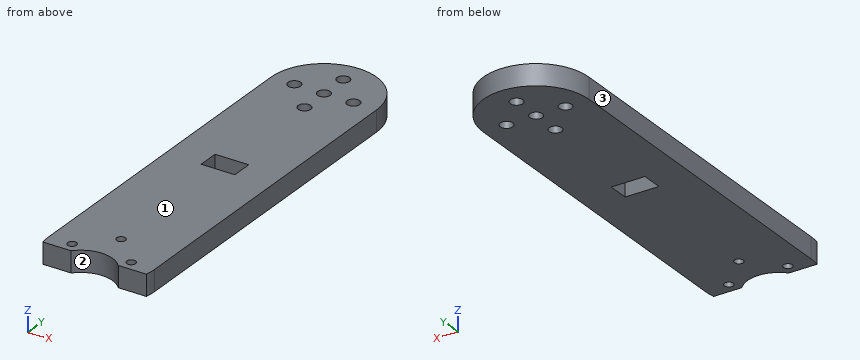
from build123d import *

# Parameters (mm, degrees)
SKETCH1_R           = 1.5
SKETCH1_R_2         = 1.493875789
SKETCH1_R_3         = 1.05
BOSS_EXTRUDE1_DEPTH = 5
SKETCH3_W           = 8
SKETCH3_H           = 5
CUT_EXTRUDE3_DEPTH  = 10
SKETCH5_R           = 7.5
SKETCH5_W           = 24.494897428
SKETCH5_H           = 10
CUT_EXTRUDE4_DEPTH  = 10


with BuildPart() as part:
    # Sketch1 → Boss-Extrude1 (new body)
    with BuildSketch(Plane.XY):
        with BuildLine():
            Line((-12.5, 0), (-12.5, -80))
            ThreePointArc((-12.5, -80), (0, -92.5), (12.5, -80))
            Line((12.5, -80), (12.5, 0))
            ThreePointArc((12.5, 0), (0, 12.5), (-12.5, 0))
        make_face()
        with Locations((0, 6.993875789)):
            Circle(SKETCH1_R, mode=Mode.SUBTRACT)
        Circle(SKETCH1_R_2, mode=Mode.SUBTRACT)
        with Locations((-7, -80)):
            Circle(SKETCH1_R_3, mode=Mode.SUBTRACT)
        with Locations((0, -73)):
            Circle(SKETCH1_R_3, mode=Mode.SUBTRACT)
        with Locations((7, -80)):
            Circle(SKETCH1_R_3, mode=Mode.SUBTRACT)
        with Locations((-6.993875789, 0)):
            Circle(SKETCH1_R, mode=Mode.SUBTRACT)
        with Locations((0, -6.993875789)):
            Circle(SKETCH1_R, mode=Mode.SUBTRACT)
        with Locations((6.993875789, 0)):
            Circle(SKETCH1_R, mode=Mode.SUBTRACT)
    extrude(amount=BOSS_EXTRUDE1_DEPTH)

    # Sketch3 → Cut-Extrude3 (cut)
    with BuildSketch(Plane.XY.offset(5)):
        with Locations((0, -35.613875789)):
            Rectangle(SKETCH3_W, SKETCH3_H)
    extrude(amount=-CUT_EXTRUDE3_DEPTH, mode=Mode.SUBTRACT)

    # Sketch5 → Cut-Extrude4 (cut)
    with BuildSketch(Plane.XY.offset(5)):
        with Locations((0, -87.5)):
            Circle(SKETCH5_R)
        with Locations((0, -87.5)):
            Rectangle(SKETCH5_W, SKETCH5_H)
    extrude(amount=-CUT_EXTRUDE4_DEPTH, mode=Mode.SUBTRACT)


solid = part.part
For this review, take the finished solid that the model builds, in its own axes (mm). Face numbers are marked on the shaded views. Give positions to 0.01 mm unless a question says otherwise; leave off trailing zeros. Loops run counter-clockwise (first coordinate to the right, second up) from the corner with the lowest first, then second, coordinate; pieces in that order, holes last.
Item 1: Take a section at C-C, the plane z = 3.3. Give the number of separate pieces and of enclosed holes in the cut face, and give its area (3 significant figures).
Item 2: Draft analysis for pull direction X (two halves, no side actions). For the marked faces 1, 2 and 3, state which applies: +X half, -X half, draft (parallel to the pull), parting line (faces both ways), or undercut.
Item 3: Take a section at D-D, the plane x = -11. State the section outline as (y, z) points.
Item 4: For line 1 along Y through (x, z) = (0, 3.45); line 2 along X through (y, z) = (-73, 3.05); line 3 along Y through (x, z) = (-0.75, 4.15), list the stretches that pass through material, from the lowest coordinate up.
Item 5: Take a section at A-A, the plane x = 0. State the section outline as (y, z) points, and give its area (3 significant figures).
Item 6: Take a section at B-B, the plane x = -7. State the section outline as (y, z) points.
Calculated:
1. separate pieces: 1
1. enclosed holes: 9
1. area: 2,200 mm2
2. face 1: draft
2. face 2: undercut
2. face 3: -X half
3. outline: (-82.5, 0) - (5.94, 0) - (5.94, 5) - (-82.5, 5) - close
4. line 1: y = -80 to -74.05, -71.95 to -38.11, -33.11 to -8.49, -5.49 to -1.49, 1.49 to 5.49, 8.49 to 12.5
4. line 2: x = -12.5 to -1.05, 1.05 to 12.5
4. line 3: y = -80.04 to -73.73, -72.27 to -38.11, -33.11 to -8.29, -5.69 to -1.29, 1.29 to 5.69, 8.29 to 12.48
5. outline: (-80, 0) - (-74.05, 0) - (-74.05, 5) - (-80, 5) - close; (-71.95, 0) - (-38.11, 0) - (-38.11, 5) - (-71.95, 5) - close; (-33.11, 0) - (-8.49, 0) - (-8.49, 5) - (-33.11, 5) - close; (-5.49, 0) - (-1.49, 0) - (-1.49, 5) - (-5.49, 5) - close; (1.49, 0) - (5.49, 0) - (5.49, 5) - (1.49, 5) - close; (8.49, 0) - (12.5, 0) - (12.5, 5) - (8.49, 5) - close
5. area: 382 mm2
6. outline: (-82.5, 0) - (-81.05, 0) - (-81.05, 5) - (-82.5, 5) - close; (-78.95, 0) - (-1.5, 0) - (-1.5, 5) - (-78.95, 5) - close; (1.5, 0) - (10.36, 0) - (10.36, 5) - (1.5, 5) - close
